Source: CAD feature listing. Evaluate the final solid. Frame: model axes, mm. A direction names the side the tool comes from. Give positions to 0.01 mm unless a question says otherwise; leave off trailing zeros. Loops run counter-clockwise (first coordinate to the right, second up) from the corner with the lowest first, then second, coordinate; pieces in that order, holes last.
from build123d import *

# Parameters (mm, degrees)
SKETCH1_R           = 15
BOSS_EXTRUDE1_DEPTH = 1000
SKETCH2_R           = 20
BOSS_EXTRUDE2_DEPTH = 70
SKETCH3_R           = 15
BOSS_EXTRUDE3_DEPTH = 45
SKETCH4_R           = 20
BOSS_EXTRUDE4_DEPTH = 70
SKETCH5_R           = 15
BOSS_EXTRUDE5_DEPTH = 45


with BuildPart() as part:
    # Sketch1 → Boss-Extrude1 (new body)
    with BuildSketch(Plane.XY):
        Circle(SKETCH1_R)
    extrude(amount=BOSS_EXTRUDE1_DEPTH)

    # Sketch2 → Boss-Extrude2 (add)
    with BuildSketch(Plane.XY.offset(1000)):
        Circle(SKETCH2_R)
    extrude(amount=BOSS_EXTRUDE2_DEPTH)

    # Sketch3 → Boss-Extrude3 (add)
    with BuildSketch(Plane.XY.offset(1070)):
        Circle(SKETCH3_R)
    extrude(amount=BOSS_EXTRUDE3_DEPTH)

    # Sketch4 → Boss-Extrude4 (add)
    with BuildSketch(Plane(origin=(0, 0, 0), x_dir=(-1, 0, 0), z_dir=(0, 0, -1))):
        Circle(SKETCH4_R)
    extrude(amount=BOSS_EXTRUDE4_DEPTH)

    # Sketch5 → Boss-Extrude5 (add)
    with BuildSketch(Plane(origin=(0, 0, -70), x_dir=(-1, 0, 0), z_dir=(0, 0, -1))):
        Circle(SKETCH5_R)
    extrude(amount=BOSS_EXTRUDE5_DEPTH)


solid = part.part
1) Reachability of faces 1 (the cylindrical face through (14.985, 0.66, -92.185)), 2 (the flat face through (-3, 15, 0)), 3 (the cylindrical face through (-14.985, 0.66, 1092.185)), 4 (the cylindrical face through (-4.336, -19.524, 1034.51)) from +Z, -Z, +X, -X, +Y, -Y: full face, straight path, thin tool, end or side. Return the list, or none.
Checks:
face 1: -Z
face 2: none
face 3: +Z
face 4: +Z, -Z
2) Contact query for flat-ended pins moving along their axis: P1, Ø3, axis at y = 4, z = 849, coming from the -X side; P2, Ø4, axis at x = 5.5, z = 784.5, coming from the +Y side; P3, Ø12, axis at y = 8.5, z = 493.5, coming from the +X side. Output: stop coordinate, or through.
Checks:
P1: stops at x = -14.79
P2: stops at y = 14.59
P3: stops at x = 14.79
3) Pull-direction query (Z, two-part tool) for faces 5 (the flat face through (-3, 15, -70)), 6 (the flat face through (3, 15, 1000)), 7 (the cylindrical face through (4.336, -19.524, -34.51)); classes: released by +Z, released by -Z, zero draft, split by the parting line, or undercut.
Checks:
face 5: released by -Z
face 6: undercut
face 7: zero draft
4) Ray query, probe 1 along Z at (x, y) = (12.5, -11.5); probe 2 along Y at (x, z) = (-13, 1048); probe 3 along Y at (x, z) = (-7.5, 708.5). Return the intervals inside material, ascending.
Checks:
probe 1: z = -70 to 0, 1000 to 1070
probe 2: y = -15.2 to 15.2
probe 3: y = -12.99 to 12.99
5) Cut plane C-C (z = 377.5). Return loops of the section in (x, y), and give its area (3 significant figures).
Checks:
outline: circle Ø30 at (0, 0)
area: 707 mm2
6) Cut plane A-A (y = 0). Return loops of the section in (x, z).
Checks:
outline: (-20, -70) - (-15, -70) - (-15, -115) - (15, -115) - (15, -70) - (20, -70) - (20, 0) - (15, 0) - (15, 1000) - (20, 1000) - (20, 1070) - (15, 1070) - (15, 1115) - (-15, 1115) - (-15, 1070) - (-20, 1070) - (-20, 1000) - (-15, 1000) - (-15, 0) - (-20, 0) - close
